Autodesk Inventor part; units mm, degrees
ref_plane "YZ Plane" through (0, 0, 0) normal (1, 0, 0) x (0, 1, 0)
ref_plane "XZ Plane" through (0, 0, 0) normal (0, 1, 0) x (-1, 0, 0)
ref_plane "XY Plane" through (0, 0, 0) normal (0, 0, 1) x (1, 0, 0)
sketch "Esquisse4" plane through (0, 0, 0) normal (1, 0, 0) x (0, 1, 0)
  line L0 (0, 0) -> (80, 0) construction
  line L1 (0, 0) -> (0, 76) construction
  line L2 (0, 76) -> (32, 76) construction
  line L3 (32, 76) -> (80, 0) construction
  line L4 (67.3684, 0) -> (67.3684, 20) construction
  line L5 (67.3684, 20) -> (0, 20) construction
  line L6 (67.3684, 20) -> (59.3585, 32.6823)
  line L7 (0, 20) -> (0, 22)
  line L8 (59.3585, 32.6823) -> (44.3585, 32.6823)
  line L9 (44.3585, 32.6823) -> (44.3585, 20)
  line L10 (44.3585, 20) -> (46.3585, 20)
  line L11 (46.3585, 20) -> (46.3585, 32.6823) construction
  line L12 (46.3585, 32.6823) -> (46.3585, 30.6823) construction
  line L13 (46.3585, 30.6823) -> (60.6217, 30.6823) construction
  line L14 (46.3585, 30.6823) -> (46.3585, 20)
  line L15 (58.2562, 30.6823) -> (65.0029, 20)
  line L16 (60.6217, 30.6823) -> (58.9307, 29.6143) construction
  line L17 (46.3585, 30.6823) -> (58.2562, 30.6823)
  line L18 (65.0029, 20) -> (67.3684, 20)
  line L19 (0, 20) -> (44.3585, 20)
  line L20 (0, 22) -> (44.3585, 22)
  dimension "d23" = 80
  dimension "d24" = 76
  dimension "d25" = 32
  dimension "d27" = 20
  dimension "d28" = 15
  dimension "d29" = 2
  dimension "d30" = 15
  dimension "d31" = 2
  dimension "d32" = 2
  dimension "d33" = 2
revolve "Révolution2" add sketch "Esquisse4" angle 90 about axis through (0, 0, 0) along (0, 0, -1)
sketch "Esquisse9" plane through (0, 0, 22) normal (0, 0, 1) x (-0.7071, 0.7071, 0)
  circle A0 centre (0, 0) radius 44.3585
  circle A1 centre (0, 0) radius 13.5
  dimension "d35" = 27
extrude "Extrusion3" cut sketch "Esquisse9" against normal blind 10 contours A1
sketch "Esquisse14" plane through (0, 44.3585, 32.6823) normal (-1, 0, 0) x (0, 0, 1)
  line L0 (0, 0) -> (-10.6823, 0)
  line L1 (-12.6823, 20.6444) -> (-12.6823, 23.0099)
  line L2 (-2, 13.8977) -> (-12.6823, 20.6444)
  line L3 (-2, 2) -> (-2, 13.8977)
  line L4 (-12.6823, -30.8585) -> (-12.6823, 2)
  line L5 (-12.6823, 20.6444) -> (-2, 13.8977)
  line L6 (-2, 13.8977) -> (-2, 0)
  line L7 (-2, 0) -> (-12.6823, 0)
  line L8 (-12.6823, 0) -> (-12.6823, 20.6444)
  point P0 (-32.6823, -44.3585)
extrude "Extrusion8" add sketch "Esquisse14" against normal blind 2
sketch "Esquisse15" plane through (44.3585, 0, 32.6823) normal (0, -1, 0) x (1, 0, 0)
  line L0 (-30.8585, -10.6823) -> (-30.8585, -12.6823)
  line L1 (-30.8585, -12.6823) -> (2, -12.6823)
  line L2 (13.8977, -2) -> (20.6444, -12.6823)
  line L3 (0, 0) -> (0, -10.6823)
  line L4 (0, -10.6823) -> (-30.8585, -10.6823)
  line L5 (20.6444, -12.6823) -> (13.8977, -2)
  line L6 (13.8977, -2) -> (0, -2)
  line L7 (0, -2) -> (0, -12.6823)
  line L8 (0, -12.6823) -> (20.6444, -12.6823)
  point P0 (-44.3585, -32.6823)
extrude "Extrusion9" add sketch "Esquisse15" against normal blind 2
sketch "Esquisse17" plane through (44.3585, 0, 32.6823) normal (0, -1, 0) x (1, 0, 0)
  line L0 (-30.8585, -12.6823) -> (23.0099, -12.6823)
  line L1 (15, 0) -> (0, 0)
  line L2 (15, 0) -> (0, 0) construction
  line L3 (7.5, 0) -> (7.5, -12.6823) construction
  circle A0 centre (7.5, -6.3412) radius 1
  point P0 (-44.3585, -32.6823)
  dimension "d61" = 2
extrude "Extrusion10" cut sketch "Esquisse17" against normal blind 2
sketch "Esquisse18" plane through (0, 44.3585, 32.6823) normal (-1, 0, 0) x (0, 0, 1)
  line L0 (-12.6823, -30.8585) -> (-12.6823, 23.0099)
  line L1 (0, 15) -> (0, 0)
  line L2 (0, 0) -> (0, 15) construction
  line L3 (0, 7.5) -> (-12.6823, 7.5) construction
  circle A0 centre (-6.3412, 7.5) radius 1
  point P0 (-32.6823, -44.3585)
  dimension "d64" = 2
extrude "Extrusion11" cut sketch "Esquisse18" against normal blind 2
sketch "Esquisse19" plane through (0, 44.3585, 32.6823) normal (0, 0, 1) x (1, 0, 0)
  arc A0 (44.3585, -44.3585) -> (0, 0) centre (0, -44.3585) ccw
  line L0 (59.3585, -44.3585) -> (44.3585, -44.3585)
  arc A1 (59.3585, -44.3585) -> (0, 15) centre (0, -44.3585) ccw
  line L1 (0, -44.3585) -> (59.3585, -44.3585) construction
  line L2 (44.3585, -44.3585) -> (59.3585, -44.3585) construction
  line L3 (0, -44.3585) -> (50.0625, -12.4652) construction
  line L4 (37.4116, -20.5247) -> (50.0625, -12.4652) construction
  circle A2 centre (43.737, -16.495) radius 2.5
  circle A3 centre (29.7448, -1.8785) radius 2.5
  circle A4 centre (11.2242, 6.2707) radius 2.5
  circle A5 centre (-9.0051, 6.7122) radius 2.5
  circle A6 centre (-27.8636, -0.6215) radius 2.5
  circle A7 centre (-42.48, -14.6137) radius 2.5
  circle A8 centre (-50.6293, -33.1343) radius 2.5
  circle A9 centre (-51.0707, -53.3637) radius 2.5
  circle A10 centre (-43.737, -72.2221) radius 2.5
  circle A11 centre (-29.7448, -86.8385) radius 2.5
  circle A12 centre (-11.2242, -94.9878) radius 2.5
  circle A13 centre (9.0051, -95.4292) radius 2.5
  circle A14 centre (27.8636, -88.0956) radius 2.5
  circle A15 centre (42.48, -74.1034) radius 2.5
  circle A16 centre (50.6293, -55.5828) radius 2.5
  circle A17 centre (51.0707, -35.3534) radius 2.5
  dimension "d67" = 32.5
  dimension "d68" = 5
  dimension "d71" = 360
extrude "Extrusion12" cut sketch "Esquisse19" against normal through all contours A2 | A3 | A4 | A17
properties part number "led"
Could you check a few things on this model? Use its own coordinates, in mm. A direction names the side the tool comes from. Give positions to 0.01 mm unless a question says otherwise; leave off trailing zeros.
1. Will these pins go through, and if not, where does the flat tip stop? P1, Ø4, axis at y = 26, z = 24, coming from the +X side; P2, Ø1, axis at y = 14.5, z = 27.5, coming from the +X side; P3, Ø1.6, axis at x = 51.86, z = 26.34, coming from the -Y side.
2. We'd pull the mould along Y, two halves only. Please class faces 1 (the flat face through (27, 26, 20)), 2 (the cylindrical face through (0.986, 51.475, 27.265)), 3 (the cylindrical face through (9.65, 9.44, 21.01)): pulls with the +Y half, pulls with the -Y half, needs draft (parallel to the pull), parting line crosses it, or undercut.
3. I need wall thicknesses on L1, parallel to Z at x = 5, y = 27; L2, parallel to X at y = 50, z = 22.5; L3, parallel to Y at x = 29.5, z = 21.75. Which ranges of each line are inside material? Lowest first, please.
4. For faces 4 (the cylindrical face through (27.76, 40.96, 31.7)), 5 (the cylindrical face through (32.44, 33.12, 25.27)), 6 (the cylindrical face through (51.121, 0.986, 27.017)), 7 (the flat face through (52, 0, 25)), 8 (the flat face through (22, 22, 22)), which set-ups out of +Z, -Z, +X, -X, +Y, -Y let a thin tool reach every point of the face, with its end or its side?
Solved:
1. P1: stops at x = 61.01
1. P2: stops at x = 61.28
1. P3: stops at y = 30.46
2. face 1: needs draft
2. face 2: undercut
2. face 3: pulls with the -Y half
3. L1: z = 20 to 22
3. L2: x = 0 to 2, 39.02 to 42.76
3. L3: y = 0 to 35.76, 56.68 to 59.33
4. face 4: +Z, -Z
4. face 5: -Z
4. face 6: -Y
4. face 7: +Z, -Z, +X, -X, -Y
4. face 8: +Z, -X, -Y
